Geometry check sheet. Reference: drawing and pictorial views, mm from the part's lowest x, y, z. Give positions to 0.01 mm unless a question says otherwise; leave off trailing zeros. Order: outer loops, then holes, each group sorted by start corner. A loop starts at its lowest first (then second) coordinate and runs counter-clockwise, first axis right, second up.
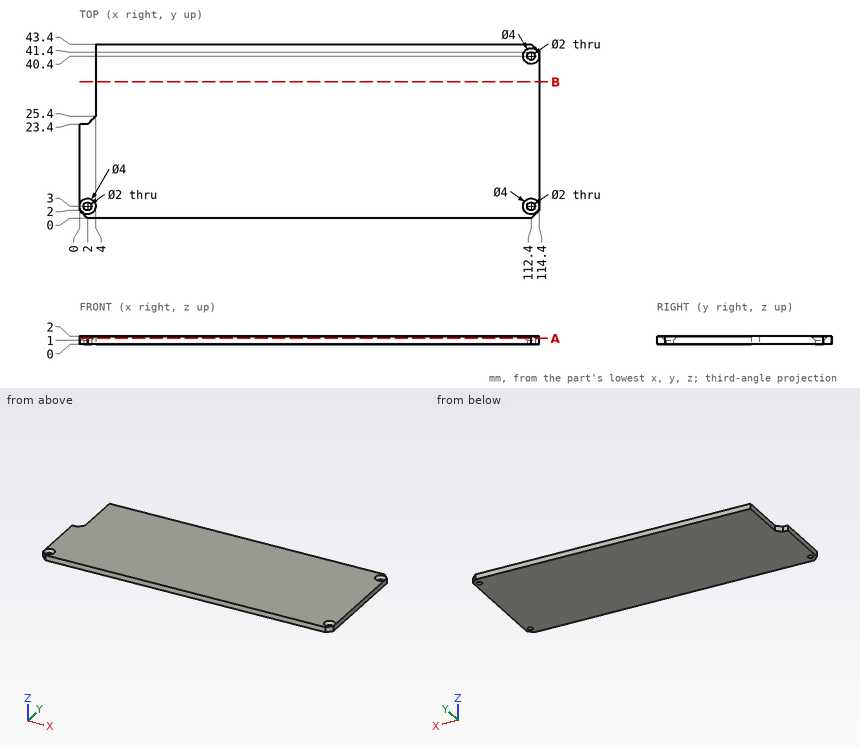
(1) Sectioned sample at B-B (y = 34). Enter the section's corners in (x, z), plus the area to 3 significant figures.
(2) Thickness scan on L1, parallel to Y at x = 112.4, z = 0.35; L2, parallel to Y at x = 2, z = 0.6; L3, parallel to X at y = 3, z = 0.3. Record the ranges inside material, lowest first.
(3) Sectioned sample at A-A (z = 1.5). Enter the section's corners in (x, y), plus the area to 3 significant figures.
(4) Go/stop test with flat-tipped pins: P1, Ø2.5, axis at x = 112.4, y = 40.4, coming from the +Z side; P2, Ø3, axis at x = 112.4, y = 3, coming from the +Z side. Record where each tip stops, or that it passes through.
Values follow:
1. outline: (4, 0) - (114.4, 0) - (114.4, 2) - (4, 2) - close
1. area: 221 mm2
2. L1: y = 0 to 2, 4 to 39.4, 41.4 to 43.4
2. L2: y = 0 to 2, 4 to 23.4
2. L3: x = 0 to 1, 3 to 111.4, 113.4 to 114.4
3. outline: (0, 2) - (2, 0) - (112.4, 0) - (114.4, 2) - (114.4, 41.4) - (112.4, 43.4) - (4, 43.4) - (4, 25.4) - (2, 23.4) - (0, 23.4) - close; hole circle Ø3 at (2, 3); hole circle Ø3 at (112.4, 3); hole circle Ø3 at (112.4, 40.4)
3. area: 4,860 mm2
4. P1: stops at z = 1.25
4. P2: stops at z = 1.5
